Can you work these out from the model? Positions are in its coordinate system, mm. Face numbers are marked on the shaded views. A direction names the side the tool comes from. Give positions to 0.01 mm unless a question says otherwise; leave off trailing zeros. Write each loop counter-clockwise with the first axis right and the second up, starting at its lowest first coordinate (ties: lowest second). Pieces come first, ordered by that corner, then holes. Notation, with made-up numbers: M 40,-25 L 74,-25 A23 ccw 74,14 Z; hole C 82,-31.75 d8. An arc over 180 degrees is marked long. Use CSV: the item, a comma, the result in double quotes. Start each with the question number.
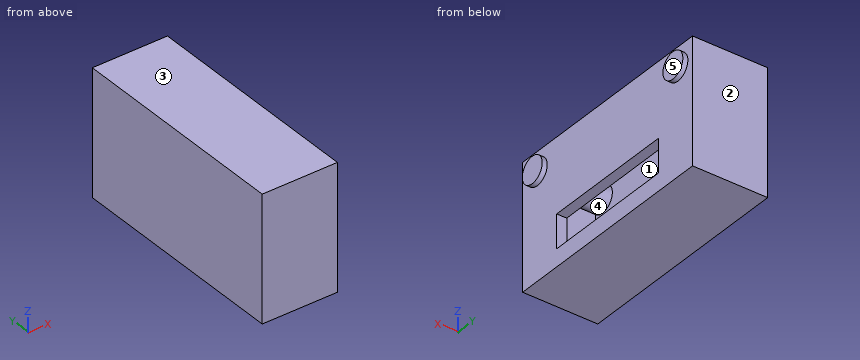
from build123d import *

# Parameters (mm, degrees)
F0_W     = 45
F0_H     = 25
F1_DEPTH = 15
F2_W     = 3.8793105632
F2_H     = 6.7036496475
F2_W_2   = 5.8189658448
F2_W_3   = 7.5361132622
F3_DEPTH = 25
F4_T     = 2
F5_R     = 2.6382169245
F6_DEPTH = 5
F7_DEPTH = 16


# Not quite as in the source:
# - a shell that OpenCascade refuses in one call is made with other operations: the cavity is built on its own and cut out


with BuildPart() as f1:
    # F0 (on Right) → F1 (new body)
    with BuildSketch(Plane.YZ):
        Rectangle(F0_W, F0_H)
    extrude(amount=F1_DEPTH)

    # F2 (on Right) → F3 (join)
    with BuildSketch(Plane.YZ):
        with Locations((-11.5266777575, -5.6595918722)):
            Rectangle(F2_W, F2_H)
        with Locations((-6.6775395535, -5.6595918722)):
            Rectangle(F2_W_2, F2_H)
        with Locations((0, -5.6595918722)):
            Rectangle(F2_W_3, F2_H)
        with Locations((6.6775395535, -5.6595918722)):
            Rectangle(F2_W_2, F2_H)
        with Locations((11.5266777575, -5.6595918722)):
            Rectangle(F2_W, F2_H)
    extrude(amount=F3_DEPTH)

    # F4: shell of thickness 2, made by hand


with BuildPart() as f4_core1:
    # F4_t2: copy of F1
    add(f1.part)

    # the walls: a layer under each face that stays
    f4_faces = [f4_core1.faces().sort_by_distance(p)[0] for p in [
        (7.5, -22.5, 0),
        (7.5, 0, 12.5),
        (7.5, 0, -12.5),
        (0, 0, 0),
        (15, 0, 0),
        (7.5, 22.5, 0),
    ]]
    thicken(f4_faces, amount=-F4_T, mode=Mode.SUBTRACT)


with BuildPart() as f1_1:
    add(f1.part)

    # what is left inside the walls is the cavity
    f4_cavity = [f4_core1.part.solids().sort_by_distance(p)[0] for p in [
        (2.02, 0, -3.5),
    ]]
    add(f4_cavity, mode=Mode.SUBTRACT)

    # F5 (on Right) → F6 (join)
    with BuildSketch(Plane.YZ):
        with Locations((-18.6206903309, 8.5344836116)):
            Circle(F5_R)
        with Locations((18.6206903309, 8.5344836116)):
            Circle(F5_R)
    extrude(amount=F6_DEPTH)

    # F5 (on Right) → F7 (join)
    with BuildSketch(Plane.YZ):
        with Locations((-18.6206903309, 8.5344836116)):
            Circle(F5_R)
        with Locations((18.6206903309, 8.5344836116)):
            Circle(F5_R)
    extrude(amount=F7_DEPTH)


solid = f1_1.part
(1) Thinking about a two-plate mould opening in Z: for the marked faces 1, 2 and 3, which applies, released by +Z, released by -Z, zero draft, split by the parting line, or undercut?
(2) I want a section at A-A (y = 14.5). Write out the boundary of the cut face in (x, z), and give its area (3 significant figures).
(3) I want a section at C-C (z = 7.5). Write out the boundary of the cut face in (x, y).
(4) I want a section at B-B (x = 13.75). Write out the boundary of the cut face in (y, z), and give its area (3 significant figures).
(5) Will these pins go through, and if not, where does the flat tip stop? pin 1 Ø6 at (y, z) = (12, 1.5) entering from -X; pin 2 Ø6.5 at (y, z) = (-1.5, 3.5) entering from +X.
(6) Which directions (+Z, -Z, +X, -X, +Y, -Y) give clear straight access to the entire face, cutting with the end or side of a thin tool? Please do the marked faces 4 and 5.
(7) I want a section at D-D (x = 10.75). Write out the boundary of the cut face in (y, z).
(8) Please list where these lines run through material, in increasing order: L1, parallel to Y at x = 11.25, z = -1; L2, parallel to X at y = -9, z = -1; L3, parallel to Z at x = 5.5, y = 7.5. Write a range as [from, to].
Geometry results:
1,face 1,"undercut"
1,face 2,"zero draft"
1,face 3,"released by +Z"
2,outline,"M 0,-12.5 L 15,-12.5 L 15,12.5 L 0,12.5 Z; hole M 2,-10.5 L 13,-10.5 L 13,10.5 L 2,10.5 Z"
2,area,"144 mm2"
3,outline,"M 0,-22.5 L 15,-22.5 L 15,-21.05 L 16,-21.05 L 16,-16.19 L 15,-16.19 L 15,16.19 L 16,16.19 L 16,21.05 L 15,21.05 L 15,22.5 L 0,22.5 Z; hole M 2,-16.19 L 13,-16.19 L 13,16.19 L 2,16.19 Z"
4,outline,"M -22.5,-12.5 L 22.5,-12.5 L 22.5,12.5 L -22.5,12.5 Z; hole M -13.47,-9.01 L 13.47,-9.01 L 13.47,-2.31 L -13.47,-2.31 Z"
4,area,"944 mm2"
5,pin 1,"stops at x = 0"
5,pin 2,"stops at x = 15"
6,face 4,"none"
6,face 5,"+Z, -Z, +X, +Y, -Y"
7,outline,"M -22.5,-12.5 L 22.5,-12.5 L 22.5,12.5 L -22.5,12.5 Z; hole M -20.5,-10.5 L 20.5,-10.5 L 20.5,6.68 A2.64 cw long 16.86,10.5 L -16.86,10.5 A2.64 cw long -20.5,6.68 Z; hole M -20.5,10.39 A2.64 cw -20.38,10.5 L -20.5,10.5 Z; hole M 20.38,10.5 A2.64 cw 20.5,10.39 L 20.5,10.5 Z"
8,L1,"y = [-22.5, -20.5], [20.5, 22.5]"
8,L2,"x = [0, 2], [13, 15]"
8,L3,"z = [-12.5, -10.5], [10.5, 12.5]"
